Build history of the part. All positions in model axes, mm. A direction names the side the tool comes from. Give positions to 0.01 mm unless a question says otherwise; leave off trailing zeros. Write each loop counter-clockwise with the first axis right and the second up, starting at its lowest first coordinate (ties: lowest second). Pieces come first, ordered by that corner, then holes. Notation, with made-up numbers: (22, -29) -> (47, -29) arc R22 cw to (47, -12) -> close; hole circle Ø10 at (-18, 10). An arc over 180 degrees is marked (long way). Put each result on its own line as item: value. Start each with the question number.
Item 1: Slice it at D-D, the plane z = -44.5. List the corners of the cut face in (x, y), plus the area to 3 significant figures.
Item 2: Slice it at B-B, the plane y = 14. List the corners of the cut face in (x, z).
Item 3: Drill centre lines: line 1 along Z through (x, y) = (0, 10.5); line 2 along Z through (x, y) = (0, 4.75); line 3 along X through (y, z) = (11, -42.5). Where is each one in solid material? Low to high.
Item 4: Slice it at C-C, the plane z = 0. List the corners of the cut face in (x, y).
Item 5: Flat gauge pins, fed straight in: pin 1 Ø4 at (y, z) = (4.5, 3) entering from +X; pin 2 Ø9.5 at (x, z) = (0, -42.5) entering from -Y; pin 3 Ø1.8 at (y, z) = (2.5, -32.5) entering from +X; pin 4 Ø3 at (y, z) = (6.5, 31) entering from -X. Where does each tip first touch, or does it go through?
Item 6: Two-plate mould, pull along Z, no slides. Class faces 5 (the flat face through (0, 0, 1)), 6 (the cylindrical face through (0.264, 2.958, 54.497)), 7 (the cylindrical face through (-0.391, 8.112, -45.474)), 8 (the flat face through (-11, 6, 1)): pulls with the +Z half, pulls with the -Z half, needs draft (parallel to the pull), parting line crosses it, or undercut.
Item 7: Tool access for faces 1 (the flat face through (-12, 3, -32)), 2 (the flat face through (-12, 3, 32)), 3 (the cylindrical face through (-1.301, 10.93, 36.643)), 4 (the flat face through (12, 3, -32)): list every direction of +Z, -Z, +X, -X, +Y, -Y with a clear straight run to the whole face (end or side of a thin tool).
Item 8: Slice it at A-A, the plane x = 0. List the corners of the cut face in (y, z).
Autodesk Inventor part; units mm, degrees
ref_plane "YZ Plane" through (0, 0, 0) normal (1, 0, 0) x (0, 1, 0)
ref_plane "XZ Plane" through (0, 0, 0) normal (0, 1, 0) x (-1, 0, 0)
ref_plane "XY Plane" through (0, 0, 0) normal (0, 0, 1) x (1, 0, 0)
sketch "Sketch1" plane through (0, 0, 0) normal (0, 1, 0) x (-1, 0, 0)
  arc A0 (12, 42.5) -> (-12, 42.5) centre (0, 42.5) ccw
  arc A1 (-12, -42.5) -> (12, -42.5) centre (0, -42.5) ccw
  line L0 (0, 42.5) -> (12, 42.5) construction
  line L1 (0, -42.5) -> (12, -42.5) construction
  line L2 (0, -42.5) -> (-12, -42.5) construction
  line L3 (0, 42.5) -> (-12, 42.5) construction
  line L4 (12, 42.5) -> (12, 21.9317)
  line L5 (12, -42.5) -> (12, -21.9317)
  line L6 (-12, -42.5) -> (-12, -21.9317)
  line L7 (-12, 42.5) -> (-12, 21.9317)
  arc A2 (-12, 21.9317) -> (-12, -21.9317) centre (0, 0) ccw
  arc A3 (12, -21.9317) -> (12, 21.9317) centre (0, 0) ccw
extrude "Extrusion1" add sketch "Sketch1" along normal blind 6
sketch "Sketch2" plane through (0, 6, 0) normal (0, 1, 0) x (1, 0, 0)
  circle A0 centre (0, 0) radius 10
  circle A1 centre (0, 0) radius 19.5 construction
  arc A2 (-12, -42.5) -> (12, -42.5) centre (0, -42.5) ccw construction
  line L0 (0, -42.5) -> (0, -54.5) construction
  arc A3 (12, 42.5) -> (-12, 42.5) centre (0, 42.5) ccw construction
  line L1 (0, 42.5) -> (0, 54.5) construction
  circle A4 centre (0, -42.5) radius 6
  circle A5 centre (0, -42.5) radius 3
  circle A6 centre (0, 42.5) radius 6
  circle A7 centre (0, 42.5) radius 3
  dimension "d11" = 20
  dimension "d12" = 39
extrude "Extrusion2" add sketch "Sketch2" along normal blind 10 contours A4 | A6
sketch "Sketch3" plane through (0, 6, 42.5) normal (0, 1, 0) x (1, 0, 0)
  circle A0 centre (0, 0) radius 3
  circle A1 centre (0, 0) radius 3
  point P0 (0, 42.5)
extrude "Extrusion3" cut sketch "Sketch3" against normal blind 7
sketch "Sketch4" plane through (0, 6, -42.5) normal (0, 1, 0) x (1, 0, 0)
  circle A0 centre (0, 0) radius 3
  point P0 (0, -42.5)
extrude "Extrusion4" cut sketch "Sketch4" against normal blind 7
sketch "Sketch5" plane through (0, 6, 0) normal (0, 1, 0) x (1, 0, 0)
  circle A0 centre (0, 0) radius 10
  dimension "d23" = 20
extrude "Extrusion5" add sketch "Sketch5" along normal blind 2
fillet "Fillet1" radius 1.5 1 edges at (-10, 8, 0)
properties part number "Coperchio Superiore"
Values follow:
1. outline: (-11.83, 0) -> (-2.24, 0) -> (-2.24, 16) -> (-5.66, 16) -> (-5.66, 6) -> (-11.83, 6) -> close; (2.24, 0) -> (11.83, 0) -> (11.83, 6) -> (5.66, 6) -> (5.66, 16) -> (2.24, 16) -> close
1. area: 184 mm2
2. outline: circle Ø12 at (0, -42.5); circle Ø12 at (0, 42.5); hole circle Ø6 at (0, -42.5); hole circle Ø6 at (0, 42.5)
3. line 1: -48.5 to -45.5, -39.5 to -36.5, 36.5 to 39.5, 45.5 to 48.5
3. line 2: -54.5 to -45.5, -39.5 to 39.5, 45.5 to 54.5
3. line 3: -6 to -3, 3 to 6
4. outline: (-25, 0) -> (25, 0) -> (25, 6) -> (10, 6) -> (10, 6.5) arc R1.5 ccw to (8.5, 8) -> (-8.5, 8) arc R1.5 ccw to (-10, 6.5) -> (-10, 6) -> (-25, 6) -> close
5. pin 1: x = 24.98
5. pin 2: y = 0
5. pin 3: x = 12
5. pin 4: x = -12
6. face 5: needs draft
6. face 6: pulls with the +Z half
6. face 7: undercut
6. face 8: undercut
7. face 1: -Z, -X, +Y, -Y
7. face 2: +Z, -X, +Y, -Y
7. face 3: +Y
7. face 4: -Z, +X, +Y, -Y
8. outline: (0, -54.5) -> (6, -54.5) -> (6, -48.5) -> (16, -48.5) -> (16, -45.5) -> (0, -45.5) -> close; (0, -39.5) -> (16, -39.5) -> (16, -36.5) -> (6, -36.5) -> (6, -10) -> (6.5, -10) arc R1.5 ccw to (8, -8.5) -> (8, 8.5) arc R1.5 ccw to (6.5, 10) -> (6, 10) -> (6, 36.5) -> (16, 36.5) -> (16, 39.5) -> (0, 39.5) -> close; (0, 45.5) -> (16, 45.5) -> (16, 48.5) -> (6, 48.5) -> (6, 54.5) -> (0, 54.5) -> close
